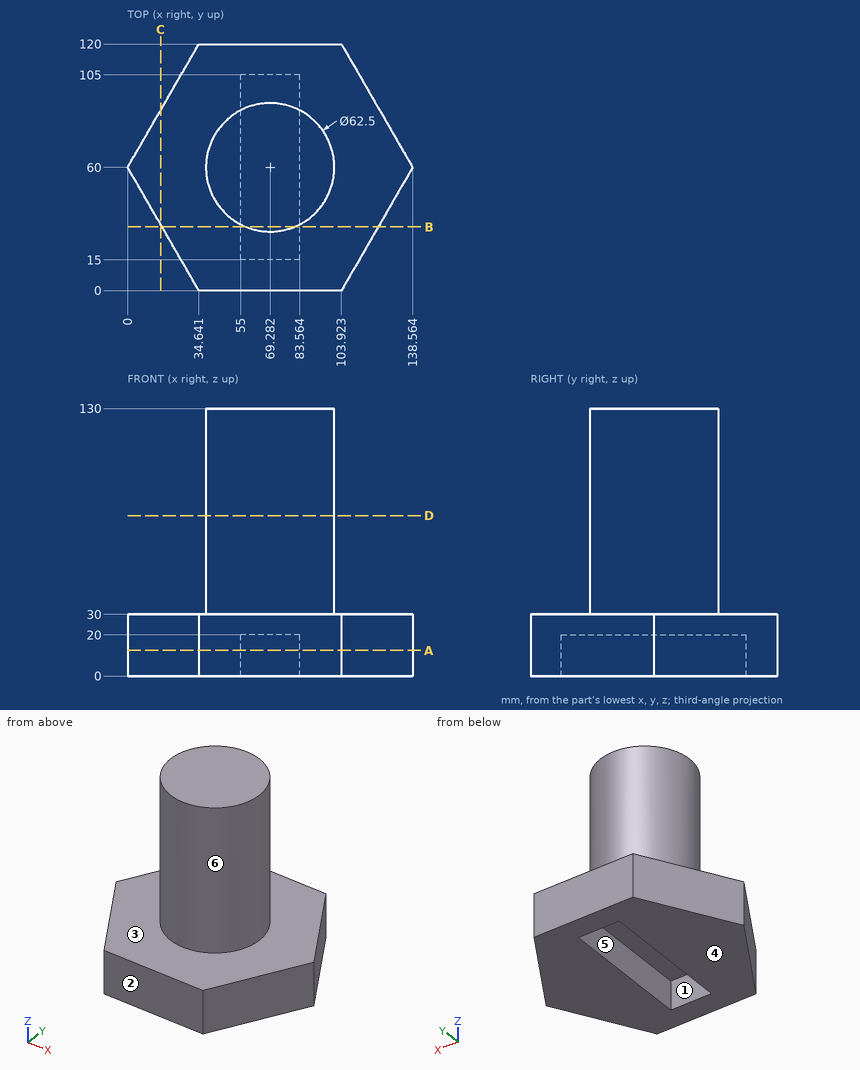
Geometry: see drawing. Coordinates: mm, zero at the bounding-box minimum. A direction names the side the tool comes from. Round coordinates to 2 decimals unless told otherwise and drop trailing zeros. Loops run counter-clockwise (first coordinate to the right, second up) from the corner with the lowest first, then second, coordinate; pieces in that order, holes last.
(1) Section query D-D (z = 78). Output: boundary loops of the cut face in (x, y).
From the geometry:
outline: circle Ø62.5 at (69.28, 60)
(2) Section query B-B (y = 31). Output: boundary loops of the cut face in (x, z).
From the geometry:
outline: (16.74, 0) - (55, 0) - (55, 20) - (83.56, 20) - (83.56, 0) - (121.82, 0) - (121.82, 30) - (80.93, 30) - (80.93, 130) - (57.64, 130) - (57.64, 30) - (16.74, 30) - close
(3) Access query for the marked faces 1, 2 and 3. Directions: +Z, -Z, +X, -X, +Y, -Y. A direction counts if a zero-diameter tool reaches every point of the face in a straight line with its end or side. Return the directions, or none.
From the geometry:
face 1: -Z
face 2: +Z, -Z, +X, -X, -Y
face 3: +Z
(4) Contact query for flat-ended pins moving along their axis: pin 1 Ø1 at (x, z) = (48.5, 83.5) entering from -Y; pin 2 Ø3 at (x, z) = (82.5, 33.5) entering from +Y; pin 3 Ø2 at (x, y) = (105, 35) entering from -Z; pin 4 Ø16 at (y, z) = (76, 12) entering from +X. Output: stop coordinate, or through.
From the geometry:
pin 1: stops at y = 36.23
pin 2: stops at y = 88.97
pin 3: stops at z = 0
pin 4: stops at x = 133.95
(5) Section query C-C (x = 16). Output: boundary loops of the cut face in (y, z).
From the geometry:
outline: (32.29, 0) - (87.71, 0) - (87.71, 30) - (32.29, 30) - close
(6) Material intervals for probe 1 along Y at (x, z) = (57.5, 13); probe 2 along Z at (x, y) = (65, 114); probe 3 along Z at (x, y) = (70.5, 83), sorted ascending.
From the geometry:
probe 1: y = 0 to 15, 105 to 120
probe 2: z = 0 to 30
probe 3: z = 20 to 130
(7) Section query A-A (z = 12.5). Output: boundary loops of the cut face in (x, y).
From the geometry:
outline: (0, 60) - (34.64, 0) - (103.92, 0) - (138.56, 60) - (103.92, 120) - (34.64, 120) - close; hole (55, 15) - (83.56, 15) - (83.56, 105) - (55, 105) - close
(8) Pull-direction query (X, two-part tool) for the marked faces 4, 5 and 6; classes: +X half, -X half, draft (parallel to the pull), parting line (faces both ways), or undercut.
From the geometry:
face 4: draft
face 5: undercut
face 6: parting line
